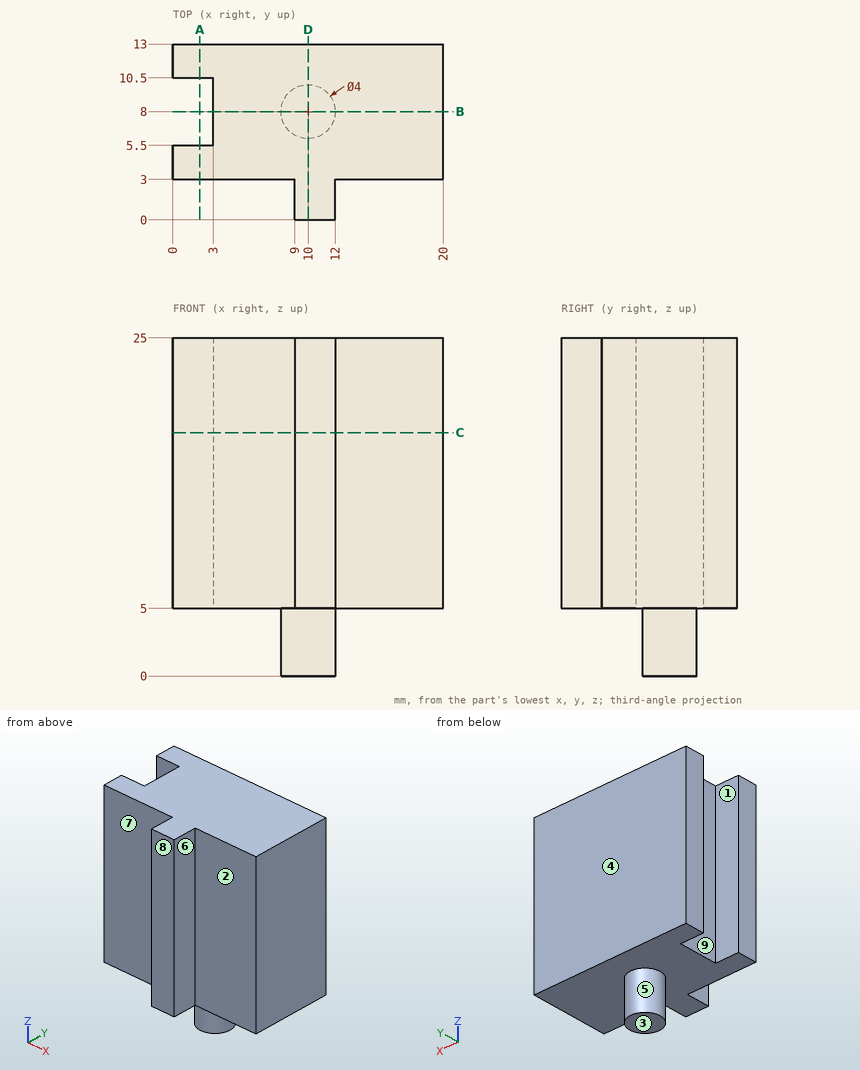
Geometry: see drawing. Coordinates: mm, zero at the bounding-box minimum. A direction names the side the tool comes from. Coordinates: 2 decimals unless noted, no trailing zeros. Loops run counter-clockwise (first coordinate to the right, second up) from the corner with the lowest first, then second, coordinate; pieces in that order, holes last. Notation, with made-up numbers: M -18.5,87.5 L 19.5,87.5 A13 cw 19.5,104.5 Z; hole C 39.25,67.5 d11. An arc over 180 degrees is marked long. Answer in a Markdown table with one row per item.
Q1. Section C-C on z = 18. Return the cut outline in (x, y), plus the area to 3 significant figures.
Answers below:
| item | result |
|---|---|
| outline | M 0,3 L 9,3 L 9,0 L 12,0 L 12,3 L 20,3 L 20,13 L 0,13 L 0,10.5 L 3,10.5 L 3,5.5 L 0,5.5 Z |
| area | 194 mm^2 |
Q2. Set-up query: the marked faces 5, 6, 7, 8 and 9. Return all of +Z, -Z, +X, -X, +Y, -Y with unobstructed straight access to the full face (end or side cutting, diameter ignored); none if empty.
Answers below:
| item | result |
|---|---|
| face 5 | -Z |
| face 6 | +Z, -Z, +X, -Y |
| face 7 | +Z, -Z, -X, -Y |
| face 8 | +Z, -Z, +X, -X, -Y |
| face 9 | +Z, -Z, -X |
Q3. Section A-A on x = 2. Return the cut outline in (y, z), plus the area to 3 significant figures.
Answers below:
| item | result |
|---|---|
| outline | M 3,5 L 5.5,5 L 5.5,25 L 3,25 Z; M 10.5,5 L 13,5 L 13,25 L 10.5,25 Z |
| area | 100 mm^2 |
Q4. Ray query, probe 1 along X at (y, z) = (1, 10.25); probe 2 along Z at (x, y) = (5.25, 7.5); probe 3 along Y at (x, z) = (13, 23.25). Return the intervals inside material, ascending. Write a range as from..to.
Answers below:
| item | result |
|---|---|
| probe 1 | x = 9..12 |
| probe 2 | z = 5..25 |
| probe 3 | y = 3..13 |
Q5. Section D-D on x = 10. Return the cut outline in (y, z), plus the area to 3 significant figures.
Answers below:
| item | result |
|---|---|
| outline | M 0,5 L 6,5 L 6,0 L 10,0 L 10,5 L 13,5 L 13,25 L 0,25 Z |
| area | 280 mm^2 |
Q6. Section B-B on y = 8. Return the cut outline in (x, z).
Answers below:
| item | result |
|---|---|
| outline | M 3,5 L 8,5 L 8,0 L 12,0 L 12,5 L 20,5 L 20,25 L 3,25 Z |
Q7. Draft query along Y for the marked faces 1, 2, 3 and 4. Return one class per face: pulls with the +Y half, pulls with the -Y half, needs draft (parallel to the pull), parting line crosses it, or undercut.
Answers below:
| item | result |
|---|---|
| face 1 | undercut |
| face 2 | pulls with the -Y half |
| face 3 | needs draft |
| face 4 | pulls with the +Y half |
Q8. First-contact query: pin 1 (2.5 mm diameter, centred on x = 1, z = 19.5, fed in from -Y); pin 2 (1.5 mm diameter, centred on y = 1.5, z = 15.5, fed in from +X); pin 3 (1.5 mm diameter, centred on y = 7.5, z = 15, fed in from -X); pin 4 (6 mm diameter, centred on x = 8.5, z = 21, fed in from -Y). Flat tips, straight axial feed; report the tip coordinate or a pass-through.
Answers below:
| item | result |
|---|---|
| pin 1 | stops at y = 3 |
| pin 2 | stops at x = 12 |
| pin 3 | stops at x = 3 |
| pin 4 | stops at y = 0 |
